Read the model definition and answer for the solid it produces. Units are mm, in the model's axes. Face numbers are marked on the shaded views. A direction names the side the tool comes from. Coordinates: 2 decimals unless noted, no trailing zeros. Order: outer loops, then holes, each group sorted by start corner. A loop starts at its lowest first (then second) coordinate and runs counter-clockwise, first axis right, second up. Notation, with made-up numbers: (-9.75, -13) -> (14.25, -13) arc R14 cw to (14.25, 7) -> close; hole circle Ø7 at (-28, 1.5). An arc over 180 degrees is marked (long way). Answer in a Markdown table with one row per item.
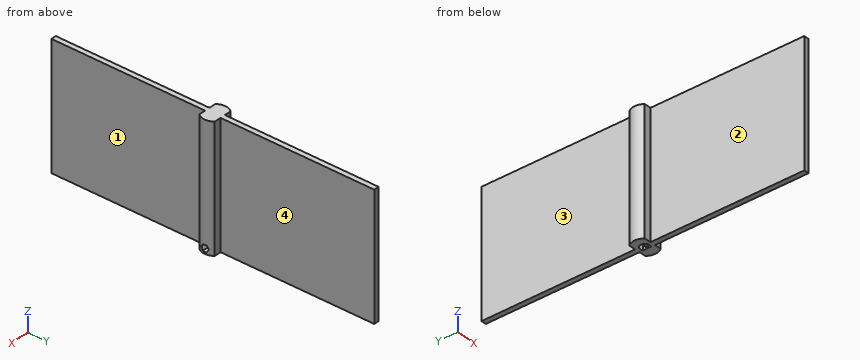
from build123d import *

# Parameters (mm, degrees)
SKETCH1_R           = 4.75
BOSS_EXTRUDE1_DEPTH = 48
CUT_EXTRUDE1_DEPTH  = 10
CUT_EXTRUDE2_DEPTH  = 49.568905691
CUT_EXTRUDE3_REACH  = 50.468
SKETCH5_W           = 2
SKETCH5_H           = 48
BOSS_EXTRUDE2_DEPTH = 60


with BuildPart() as part:
    # Sketch1 → Boss-Extrude1 (new body)
    with BuildSketch(Plane.XY):
        Circle(SKETCH1_R)
    extrude(amount=BOSS_EXTRUDE1_DEPTH)

    # Sketch2 → Cut-Extrude1 (cut)
    with BuildSketch(Plane(origin=(0, 0, 0), x_dir=(-1, 0, 0), z_dir=(0, 0, -1))):
        with BuildLine():
            Line((-0.94, 1.535057002), (-0.94, -1.535057002))
            ThreePointArc((-0.94, -1.535057002), (1.8, 0), (-0.94, 1.535057002))
        make_face()
    extrude(amount=-CUT_EXTRUDE1_DEPTH, mode=Mode.SUBTRACT)

    # Sketch3 → Cut-Extrude2 (cut, through all)
    with BuildSketch(Plane.ZY.offset(-0.94)):
        Polygon((3.230708553, 0.754115238), (1.962271323, 1.44288249), (0.73156277, 0.688767252), (0.769291447, -0.754115238), (2.037728677, -1.44288249), (3.26843723, -0.688767252), align=None)
    extrude(amount=-CUT_EXTRUDE2_DEPTH, mode=Mode.SUBTRACT)

    # Sketch4 → Cut-Extrude3 (cut, up to next)
    with BuildSketch(Plane(origin=(0, 0, 0), x_dir=(-1, 0, 0), z_dir=(0, 0, -1)), mode=Mode.PRIVATE) as cut_extrude3_sk1:
        with BuildLine():
            Line((-3.682729966, 3), (3.682729966, 3))
            ThreePointArc((3.682729966, 3), (0, 4.75), (-3.682729966, 3))
        make_face()
    cut_extrude3_tool1 = extrude(cut_extrude3_sk1.sketch, amount=-CUT_EXTRUDE3_REACH, mode=Mode.PRIVATE) & part.part
    # Sketch4 → Cut-Extrude3 (cut, up to next)
    with BuildSketch(Plane(origin=(0, 0, 0), x_dir=(-1, 0, 0), z_dir=(0, 0, -1)), mode=Mode.PRIVATE) as cut_extrude3_sk2:
        with BuildLine():
            Line((-3.682729966, -3), (3.682729966, -3))
            ThreePointArc((3.682729966, -3), (0, -4.75), (-3.682729966, -3))
        make_face()
    cut_extrude3_tool2 = extrude(cut_extrude3_sk2.sketch, amount=-CUT_EXTRUDE3_REACH, mode=Mode.PRIVATE) & part.part
    add(cut_extrude3_tool1.solids().sort_by_distance((0, 3.712383, 0))[0], mode=Mode.SUBTRACT)
    add(cut_extrude3_tool2.solids().sort_by_distance((0, -3.712383, 0))[0], mode=Mode.SUBTRACT)

    # Sketch5 → Boss-Extrude2 (add)
    with BuildSketch(Plane(origin=(0, 3, 0), x_dir=(1, 0, 0), z_dir=(0, 1, 0))):
        with Locations((0, -24)):
            Rectangle(SKETCH5_W, SKETCH5_H)
    boss_extrude2 = extrude(amount=BOSS_EXTRUDE2_DEPTH)

    # Mirror2: Boss-Extrude2 across plane
    add(boss_extrude2.mirror(Plane.ZX))


solid = part.part
Q1. Given pin 1 (5 mm diameter, centred on y = 17, z = 28, fed in from +X); pin 2 (1.5 mm diameter, centred on x = 2, z = 22.5, fed in from -Y); pin 3 (0.8 mm diameter, centred on x = 2.5, z = 13, fed in from +Y), each flat-ended and moving along its own axis, determine where each tip first touches the part or whether it passes through.
Outcome:
| item | result |
|---|---|
| pin 1 | x = 1 |
| pin 2 | y = -3 |
| pin 3 | y = 3 |
Q2. The part is cut by section A-A (x = 2.25). Write down the section's boundary in (y, z).
Outcome:
| item | result |
|---|---|
| outline | (-3, 0) -> (3, 0) -> (3, 48) -> (-3, 48) -> close; hole (-1.44, 2.04) -> (-0.75, 0.77) -> (0.69, 0.73) -> (1.44, 1.96) -> (0.75, 3.23) -> (-0.69, 3.27) -> close |
Q3. The part is cut by section B-B (z = 28). Write down the section's boundary in (x, y), then the cut area to 3 significant figures.
Outcome:
| item | result |
|---|---|
| outline | (-3.68, -3) -> (-1, -3) -> (-1, -63) -> (1, -63) -> (1, -3) -> (3.68, -3) arc R4.75 ccw to (3.68, 3) -> (1, 3) -> (1, 63) -> (-1, 63) -> (-1, 3) -> (-3.68, 3) arc R4.75 ccw to start |
| area | 293 mm² |
Q4. The part is cut by section C-C (y = 45). Write down the section's boundary in (x, z), then the cut area to 3 significant figures.
Outcome:
| item | result |
|---|---|
| outline | (-1, 0) -> (1, 0) -> (1, 48) -> (-1, 48) -> close |
| area | 96.0 mm² |
Q5. Consider line 1 (Y direction, x = 0, z = 8.25); line 2 (X direction, y = -4, z = 29); line 3 (Y direction, x = 3, z = 12). Determine where each line is inside the solid, lowest interval first.
Outcome:
| item | result |
|---|---|
| line 1 | -63 to -1.8, 1.8 to 63 |
| line 2 | -1 to 1 |
| line 3 | -3 to 3 |
Q6. For the marked faces 1, 2, 3 and 4, determine the directions among +Z, -Z, +X, -X, +Y, -Y from which every point of the face is accessible in a straight line to the end or side of a thin tool.
Outcome:
| item | result |
|---|---|
| face 1 | +Z, -Z, +X, -Y |
| face 2 | +Z, -Z, -X, -Y |
| face 3 | +Z, -Z, -X, +Y |
| face 4 | +Z, -Z, +X, +Y |
